Read the model definition and answer for the solid it produces. Units are mm, in the model's axes. Give positions to 0.01 mm unless a question says otherwise; leave off trailing zeros. Answer as CSV lines item,"result".
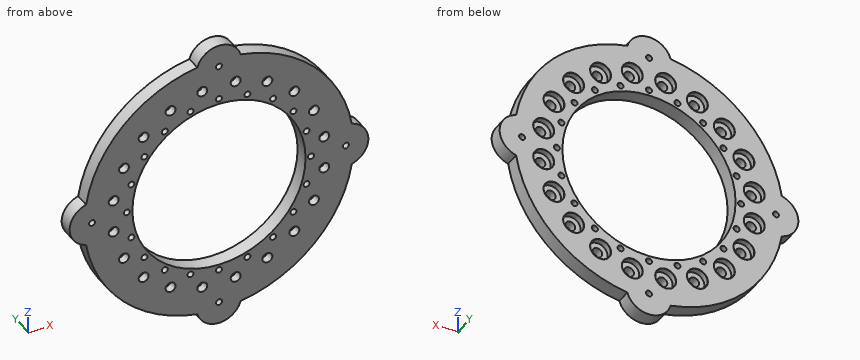
```python
from build123d import *

# Parameters (mm, degrees)
SKETCH3_R               = 114.3
SKETCH3_R_2             = 73.533
BOSS_EXTRUDE1_DEPTH     = 12.7
SKETCH16_R              = 19.05
BOSS_EXTRUDE2_DEPTH     = 12.7
CIRPATTERN6_COUNT       = 4
CIRPATTERN2_COUNT       = 20
F_1_4_20_TAPPED_HOLE2_D = 5.1054
CIRPATTERN4_COUNT       = 20
F_1_4_20_TAPPED_HOLE3_D = 5.1054


with BuildPart() as part:
    # Sketch3 → Boss-Extrude1 (new body)
    with BuildSketch(Plane(origin=(0, 0, 0), x_dir=(1, 0, 0), z_dir=(0, 1, 0))):
        Circle(SKETCH3_R)
        Circle(SKETCH3_R_2, mode=Mode.SUBTRACT)
    extrude(amount=BOSS_EXTRUDE1_DEPTH)

    # Sketch16 → Boss-Extrude2 (add)
    with BuildSketch(Plane(origin=(0, 12.7, 0), x_dir=(1, 0, 0), z_dir=(0, 1, 0))):
        with Locations((107.763073453, 0)):
            Circle(SKETCH16_R)
    boss_extrude2 = extrude(amount=-BOSS_EXTRUDE2_DEPTH)

    # CirPattern6: Boss-Extrude2 ×4 about axis
    cirpattern6_axis = Axis((0, 0, 0), (0, 1, 0))
    for i in range(1, CIRPATTERN6_COUNT):
        add(boss_extrude2.rotate(cirpattern6_axis, i * 360 / CIRPATTERN6_COUNT))

    # Sketch8 → CBORE for 5_16 Binding Head Machine Scre (revolve, cut)
    with BuildSketch(Plane(origin=(89.411079645, 12.7, -14.161323808), x_dir=(0, 0, 1), z_dir=(1, 0, 0))):
        Polygon((0, 0), (0, 12.7), (4.2164, 12.7), (4.2164, 5.3086), (8.73125, 5.3086), (8.73125, 0.15875), (8.89, 0), align=None)
    cbore_for_5_16_binding_head_machine_scre = revolve(axis=Axis((89.411079645, 19.05, -14.161323808), (0, -1, 0)), mode=Mode.SUBTRACT)

    # CirPattern2: CBORE for 5_16 Binding Head Machine Scre ×20 about axis
    cirpattern2_axis = Axis((0, 0, 0), (0, 1, 0))
    for i in range(1, CIRPATTERN2_COUNT):
        add(cbore_for_5_16_binding_head_machine_scre.rotate(cirpattern2_axis, i * 360 / CIRPATTERN2_COUNT), mode=Mode.SUBTRACT)

    # 1_4-20 Tapped Hole2 (through all)
    with Locations(Plane(origin=(0, 12.7, 0), x_dir=(1, 0, 0), z_dir=(0, 1, 0))):
        with Locations((78.232, 0)):
            f_1_4_20_tapped_hole2 = Hole(F_1_4_20_TAPPED_HOLE2_D / 2)

    # CirPattern4: 1_4-20 Tapped Hole2 ×20 about axis
    cirpattern4_axis = Axis((0, 0, 0), (0, 1, 0))
    for i in range(1, CIRPATTERN4_COUNT):
        add(f_1_4_20_tapped_hole2.rotate(cirpattern4_axis, i * 360 / CIRPATTERN4_COUNT), mode=Mode.SUBTRACT)

    # 1_4-20 Tapped Hole3 (through all)
    with Locations(Plane(origin=(0, 12.7, 0), x_dir=(1, 0, 0), z_dir=(0, 1, 0))):
        with Locations((107.763073453, 0), (0, -107.763073453), (-107.763073453, 0), (0, 107.763073453)):
            Hole(F_1_4_20_TAPPED_HOLE3_D / 2)


solid = part.part
```
(1) Find the intervals of material crossed by L1, parallel to Z at x = -74, y = 12.25; L2, parallel to X at y = 6.75, z = 12; L3, parallel to X at y = 5.5, z = 87.5, in increasing order.
Worked out:
L1,"z = -87.11 to -46.75, -35.45 to -26.7, -21.65 to 21.65, 26.7 to 35.45, 46.75 to 87.11"
L2,"x = -122.56 to -93.03, -85.79 to -72.55, 72.55 to 85.79, 93.03 to 122.56"
L3,"x = -73.54 to -17.92, -10.4 to 10.4, 17.92 to 73.54"
(2) A cutting plane is placed at A-A (z = -14). Count the separate pieces of the cut face and the enclosed holes in it, and give its area (3 significant figures).
Worked out:
separate pieces,"4"
enclosed holes,"0"
area,"922 mm^2"
(3) Each of these flat-tipped pins is pushed along its axis until it touches: P1, Ø19, axis at x = 41.5, z = 79, coming from the +Y side; P2, Ø9.5, axis at x = 41.1, z = 80.66, coming from the +Y side; P3, Ø4, axis at y = 7.5, z = -71.5, coming from the -X side; P4, Ø4.5, axis at x = -45.98, z = 63.29, coming from the +Y side. Where does it stop, or does it pass through?
Worked out:
P1,"stops at y = 12.7"
P2,"stops at y = 7.39"
P3,"stops at x = -90.74"
P4,"passes through"
